from build123d import *
from build123d.topology import SkipClean

# Parameters (mm, degrees)
SKETCH_1_R          = 28
SKETCH_1_R_2        = 2
SKETCH_1_R_3        = 21
EXTRUDE_1_DEPTH     = 2
EXTRUDE_3_DEPTH     = 30
EXTRUDE_START       = -10
SKETCH_5_R          = 28
SKETCH_5_R_2        = 21
EXTRUDE_4_DEPTH     = 10
SKETCH_6_W          = 5.360290559
SKETCH_6_H          = 32
EXTRUDE_6_DEPTH     = 100
SKETCH_9_R          = 21
CUT_EXTRUDE_1_DEPTH = 32
SKETCH_11_W         = 21.441162236
SKETCH_11_H         = 32
SKETCH_11_R         = 2
EXTRUDE_7_DEPTH     = 2
FILLET_1_R          = 3


with BuildPart() as part:
    # 草图1 → 凸台-拉伸1 (new body)
    with BuildSketch(Plane(origin=(0, 0, 0), x_dir=(1, 0, 0), z_dir=(0, 1, 0))):
        with Locations(Location((0, 0, 0), (0, 0, 270))):
            Circle(SKETCH_1_R)
        with Locations(Location((-24.5, 0, 0), (0, 0, 270))):
            Circle(SKETCH_1_R_2, mode=Mode.SUBTRACT)
        with Locations(Location((0, 24.5, 0), (0, 0, 270))):
            Circle(SKETCH_1_R_2, mode=Mode.SUBTRACT)
        with Locations(Location((24.5, 0, 0), (0, 0, 270))):
            Circle(SKETCH_1_R_2, mode=Mode.SUBTRACT)
        with Locations(Location((0, -24.5, 0), (0, 0, 270))):
            Circle(SKETCH_1_R_2, mode=Mode.SUBTRACT)
        with Locations(Location((0, 0, 0), (0, 0, 270))):
            Circle(SKETCH_1_R_3, mode=Mode.SUBTRACT)
    extrude(amount=EXTRUDE_1_DEPTH)

    # 草图2 → 凸台-拉伸3 (add)
    with SkipClean():  # the faces are left unmerged after this step: merging them gives an invalid solid
        with BuildSketch(Plane(origin=(0, 2, 0), x_dir=(1, 0, 0), z_dir=(0, 1, 0))):
            with BuildLine():
                ThreePointArc((-20.522761723, 4.451544819), (-14.849242405, 14.849242405), (-4.451544819, 20.522761723))
                Line((-4.451544819, 20.522761723), (-5.935393092, 27.363682297))
                ThreePointArc((-5.935393092, 27.363682297), (-19.798989873, 19.798989873), (-27.363682297, 5.935393092))
                Line((-27.363682297, 5.935393092), (-20.522761723, 4.451544819))
            make_face()
            with BuildLine():
                ThreePointArc((5.935393092, -27.363682297), (19.798989873, -19.798989873), (27.363682297, -5.935393092))
                Line((27.363682297, -5.935393092), (20.522761723, -4.451544819))
                ThreePointArc((20.522761723, -4.451544819), (14.849242405, -14.849242405), (4.451544819, -20.522761723))
                Line((4.451544819, -20.522761723), (5.935393092, -27.363682297))
            make_face()
            with BuildLine():
                ThreePointArc((-4.451544819, -20.522761723), (-14.849242405, -14.849242405), (-20.522761723, -4.451544819))
                Line((-20.522761723, -4.451544819), (-27.363682297, -5.935393092))
                ThreePointArc((-27.363682297, -5.935393092), (-19.798989873, -19.798989873), (-5.935393092, -27.363682297))
                Line((-5.935393092, -27.363682297), (-4.451544819, -20.522761723))
            make_face()
            with BuildLine():
                Line((4.451544819, 20.522761723), (5.935393092, 27.363682297))
                ThreePointArc((5.935393092, 27.363682297), (19.798989873, 19.798989873), (27.363682297, 5.935393092))
                Line((27.363682297, 5.935393092), (20.522761723, 4.451544819))
                ThreePointArc((20.522761723, 4.451544819), (14.849242405, 14.849242405), (4.451544819, 20.522761723))
            make_face()
        extrude(amount=EXTRUDE_3_DEPTH)

    # 草图5 → 凸台-拉伸4 (add)
    with SkipClean():  # the faces are left unmerged after this step: merging them gives an invalid solid
        with BuildSketch(Plane(origin=(0, 32, 0), x_dir=(1, 0, 0), z_dir=(0, 1, 0)).offset(EXTRUDE_START)):
            with Locations(Location((0, 0, 0), (0, 0, 270))):
                Circle(SKETCH_5_R)
            with Locations(Location((0, 0, 0), (0, 0, 270))):
                Circle(SKETCH_5_R_2, mode=Mode.SUBTRACT)
        extrude(amount=EXTRUDE_4_DEPTH)

    # 草图6 → 凸台-拉伸6 (add)
    with SkipClean():  # the faces are left unmerged after this step: merging them gives an invalid solid
        with BuildSketch(Plane(origin=(-12.25, 0, -12.25), x_dir=(-0.7071067811865488, 0, 0.7071067811865462), z_dir=(-0.7071067811865462, 0, -0.7071067811865488))):
            with Locations((-8.040435839, 16)):
                Rectangle(SKETCH_6_W, SKETCH_6_H)
            with Locations((8.040435839, 16)):
                Rectangle(SKETCH_6_W, SKETCH_6_H)
        extrude(amount=EXTRUDE_6_DEPTH)

    # 草图9 → 切除-拉伸1 (cut)
    with SkipClean():  # the faces are left unmerged after this step: merging them gives an invalid solid
        with BuildSketch(Plane.XZ):
            with Locations(Location((0, 0, 0), (0, 0, 90))):
                Circle(SKETCH_9_R)
        extrude(amount=-CUT_EXTRUDE_1_DEPTH, mode=Mode.SUBTRACT)
    add(part.part.scale(1), mode=Mode.REPLACE)  # the faces are merged on a copy

    # 草图11 → 凸台-拉伸7 (add)
    with SkipClean():  # the faces are left unmerged after this step: merging them gives an invalid solid
        with BuildSketch(Plane(origin=(-82.960678119, 0, -82.960678119), x_dir=(-0.7071067811865488, 0, 0.7071067811865462), z_dir=(-0.7071067811865462, 0, -0.7071067811865488))):
            with Locations((0, 16)):
                Rectangle(SKETCH_11_W, SKETCH_11_H)
            with Locations((0, 4)):
                Circle(SKETCH_11_R, mode=Mode.SUBTRACT)
            with Locations((0, 28)):
                Circle(SKETCH_11_R, mode=Mode.SUBTRACT)
        extrude(amount=EXTRUDE_7_DEPTH)

    # 圆角1
    fillet_1_edges = [part.edges().sort_by_distance(p)[0] for p in [
        (-15.642500311, 12, -23.223095918),
        (-23.223095918, 12, -15.642500311),
    ]]
    fillet(fillet_1_edges, radius=FILLET_1_R)


solid = part.part
Check sheet for the modelled part. Datum: model origin and axes. Units: mm. A direction names the side the tool comes from. Give positions to 0.01 mm unless a question says otherwise; leave off trailing zeros. Loops run counter-clockwise (first coordinate to the right, second up) from the corner with the lowest first, then second, coordinate; pieces in that order, holes last. Notation, with made-up numbers: M 32.5,-35 L 71.5,-35 A14 cw 71.5,-30 Z; hole C -35,-38.75 d6. An arc over 180 degrees is marked long. Return JSON: item names as keys, results as strings. Group by question number.
1. Mould release check, pull along Z, two halves, no side actions. Record for faces 1 (the flat face through (-29, 0, -20)), 2 (the cylindrical face through (22.548, 0.986, -0.434)), 3 (the flat face through (5.183, 11.86, 23.895)), 4 (the flat face through (-84.27, 16.22, -84.48)): released by +Z, released by -Z, zero draft, split by the parting line, or undercut.
2. Cross-section at D-D on z = -54. Record the boundary of the cut face in (x, y).
3. Thickness scan on L1, parallel to X at y = 1, z = 0; L2, parallel to X at y = 1.5, z = -24.5; L3, parallel to X at y = 6, z = -21. Record the ranges inside material, lowest first.
4. Cross-section at C-C on x = -65.5. Record the boundary of the cut face in (y, z).
5. Cross-section at B-B on z = 0. Record the boundary of the cut face in (x, y), plus the area to 3 significant figures.
6. Go/stop test with flat-tipped pins: pin 1 (10 mm diameter, centred on x = -65.5, y = 23, fed in from -Z); pin 2 (2 mm diameter, centred on x = -59.5, y = 4.5, fed in from -Z); pin 3 (3 mm diameter, centred on x = -24.5, z = 0, fed in from -Y). Record where each tip stops, or that it passes through.
7. Tool access check on faces 5 (the flat face through (-1.2, 2, -22.7)), 6 (the flat face through (22.7, 2, 1.2)), 7 (the cylindrical face through (-23.45, 15.78, -17.19)). Record the directions out of +Z, -Z, +X, -X, +Y, -Y that give a thin tool (end or side, any length) a straight path to the whole face; none if there is none.
8. Cross-section at A-A on y = 7.5. Record the boundary of the cut face in (x, z).
Return value:
{
 "1": {"face 1": "zero draft", "face 2": "undercut", "face 3": "released by +Z", "face 4": "released by -Z"},
 "2": {"outline": "M -69.16,0 L -61.58,0 L -61.58,32 L -69.16,32 Z; M -46.42,0 L -38.84,0 L -38.84,32 L -46.42,32 Z"},
 "3": {"L1": "-28 to -26.5, -22.5 to -21, 21 to 22.5, 26.5 to 28", "L2": "-39.66 to -32.08, -17.35 to -2, 2 to 13.56", "L3": "-36.16 to -28.58, -18.52 to -4.56, 4.56 to 18.52"},
 "4": {"outline": "M 0,-80.66 L 32,-80.66 L 32,-73.08 L 0,-73.08 Z; M 0,-57.92 L 32,-57.92 L 32,-50.34 L 0,-50.34 Z"},
 "5": {"outline": "M -28,0 L -26.5,0 L -26.5,2 L -28,2 Z; M -28,22 L -21,22 L -21,32 L -28,32 Z; M -22.5,0 L -21,0 L -21,2 L -22.5,2 Z; M 21,0 L 22.5,0 L 22.5,2 L 21,2 Z; M 21,22 L 28,22 L 28,32 L 21,32 Z; M 26.5,0 L 28,0 L 28,2 L 26.5,2 Z", "area": "152 mm^2"},
 "6": {"pin 1": "z = -85.66", "pin 2": "z = -75.66", "pin 3": "y = 22"},
 "7": {"face 5": "-Z", "face 6": "+X", "face 7": "+Y, -Y"},
 "8": {"outline": "M -91.96,-76.79 L -76.79,-91.96 L -10.71,-25.87 A28 ccw -5.94,-27.36 L -4.45,-20.52 A21 cw -20.52,-4.45 L -27.36,-5.94 A28 ccw -25.87,-10.71 Z; M -27.36,5.94 L -20.52,4.45 A21 cw -4.45,20.52 L -5.94,27.36 A28 ccw Z; M 4.45,-20.52 L 5.94,-27.36 A28 ccw 27.36,-5.94 L 20.52,-4.45 A21 cw Z; M 4.45,20.52 A21 cw 20.52,4.45 L 27.36,5.94 A28 ccw 5.94,27.36 Z; hole M -86.75,-79.17 L -79.17,-86.75 L -18.07,-25.65 A3 ccw -18.23,-21.25 A28 cw -21.25,-18.23 A3 ccw -25.65,-18.07 Z"}
}
